from build123d import *

# Parameters (mm, degrees)
SKETCH1_W           = 180
SKETCH1_H           = 75.87
SKETCH1_W_2         = 160
SKETCH1_H_2         = 2
BOSS_EXTRUDE1_DEPTH = 3


with BuildPart() as part:
    # Sketch1 → Boss-Extrude1 (new body)
    with BuildSketch(Plane(origin=(0, 0, 0), x_dir=(1, 0, 0), z_dir=(0, 1, 0))):
        with Locations((-5.566969943, 7.461475771)):
            Rectangle(SKETCH1_W, SKETCH1_H)
        with Locations((-5.566969943, 24.396475771)):
            Rectangle(SKETCH1_W_2, SKETCH1_H_2, mode=Mode.SUBTRACT)
        with Locations((-5.566969943, 32.396475771)):
            Rectangle(SKETCH1_W_2, SKETCH1_H_2, mode=Mode.SUBTRACT)
        with Locations((-5.566969943, 16.396475771)):
            Rectangle(SKETCH1_W_2, SKETCH1_H_2, mode=Mode.SUBTRACT)
        with Locations((-5.566969943, 8.396475771)):
            Rectangle(SKETCH1_W_2, SKETCH1_H_2, mode=Mode.SUBTRACT)
        with Locations((-5.566969943, 0.396475771)):
            Rectangle(SKETCH1_W_2, SKETCH1_H_2, mode=Mode.SUBTRACT)
        with Locations((-5.566969943, -7.603524229)):
            Rectangle(SKETCH1_W_2, SKETCH1_H_2, mode=Mode.SUBTRACT)
        with Locations((-5.566969943, -15.603524229)):
            Rectangle(SKETCH1_W_2, SKETCH1_H_2, mode=Mode.SUBTRACT)
    extrude(amount=BOSS_EXTRUDE1_DEPTH)


solid = part.part
The listing builds one solid part. Answer for the finished solid, in the listing's coordinates (mm). A direction names the side the tool comes from. Give positions to 0.01 mm unless a question says otherwise; leave off trailing zeros. Put each result on its own line as item: value.
Item 1: A cutting plane is placed at A-A on x = -17. Count the separate pieces of the cut face and the enclosed holes in it, plus the area to 3 significant figures.
Established:
separate pieces: 8
enclosed holes: 0
area: 186 mm^2
Item 2: For faces 5 (the face through (-7, 0, 9)), 6 (the face through (-7, 1, -1.396)), determine the directions among +Z, -Z, +X, -X, +Y, -Y from which every point of the face is accessible in a straight line to the end or side of a thin tool.
Established:
face 5: +Z, -Z, +X, -X, -Y
face 6: +Y, -Y
Item 3: For a pull along Z with two mould halves and no side action, classify faces 1 (the face through (-7, 1, -45.396)), 2 (the face through (-7, 1, 16.604)), 3 (the face through (-7, 1, 30.474)), 4 (the face through (-7, 3, 9)) as released by +Z, released by -Z, zero draft, split by the parting line, or undercut.
Established:
face 1: released by -Z
face 2: undercut
face 3: released by +Z
face 4: zero draft
